Geometry: final body of the model. Coordinates: model frame, mm. Give positions to 0.01 mm unless a question says otherwise; leave off trailing zeros. Write each loop counter-clockwise with the first axis right and the second up, starting at its lowest first coordinate (ties: lowest second). Pieces come first, ordered by that corner, then holes. Notation, with made-up numbers: M -33,25.25 L 18,25.25 A23 cw 18,33.25 Z; hole C 9.5,-22.5 d7. An arc over 180 degrees is marked long. Use a Markdown table: item, result. Add a question column.
1) Pin query (flat end, axial travel): pin 1 (1.3 mm diameter, centred on x = -10.94, y = -4.36, fed in from -Z) (3 decimals). Return the tip coordinate at first contact, or that it passes through.
2) Section D-D on y = -1.5. Return the cut outline in (x, z), then the cut area to 3 significant figures.
3) Section C-C on x = -6. Return the cut outline in (y, z).
4) Line query: line 1 (Y direction, x = -10.5, z = 0.15); line 2 (Y direction, x = -5, z = 1.5); line 3 (X direction, y = -2.75, z = 0.25). Output: solid intervals per line, ascending.
5) Section B-B on z = 2.45. Return the cut outline in (x, y), then the cut area to 3 significant figures.
6) Section A-A on x = -10.5. Return the cut outline in (y, z).
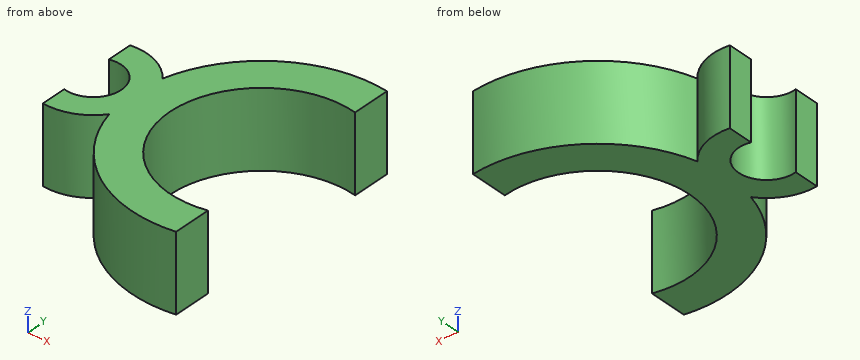
```python
from build123d import *

# Parameters (mm, degrees)
F1_DEPTH = 3


with BuildPart() as f1:
    # F0 (on Top) → F1 (new body)
    with BuildSketch(Plane.XY):
        with BuildLine():
            ThreePointArc((-3.568038, -7.869875), (-7.935237, -4.352574), (-3.568038, -0.835273))
            Line((-3.568038, -0.835273), (-3.568038, 0.689391))
            ThreePointArc((-3.568038, 0.689391), (-7.146301, -0.097234), (-9.273883, -3.079873))
            ThreePointArc((-9.273883, -3.079873), (-10.131319, -2.418957), (-11.20402, -2.272952))
            Line((-11.20402, -2.272952), (-11.20402, -3.288286))
            ThreePointArc((-11.20402, -3.288286), (-9.841317, -4.356456), (-11.20402, -5.424626))
            Line((-11.20402, -5.424626), (-11.20402, -6.439959))
            ThreePointArc((-11.20402, -6.439959), (-10.13018, -6.293478), (-9.272384, -5.631078))
            ThreePointArc((-9.272384, -5.631078), (-7.1438, -8.609565), (-3.568038, -9.394538))
            Line((-3.568038, -9.394538), (-3.568038, -7.869875))
        make_face()
    extrude(amount=F1_DEPTH)


solid = f1.part
```
Found:
| question | item | result |
|---|---|---|
| 1 | pin 1 | through |
| 2 | outline | M -8.56,0 L -6.53,0 L -6.53,3 L -8.56,3 Z |
| 2 | area | 6.09 mm² |
| 3 | outline | M -9.17,0 L -7.54,0 L -7.54,3 L -9.17,3 Z; M -1.16,0 L 0.47,0 L 0.47,3 L -1.16,3 Z |
| 4 | line 1 | -6.41 to -5.36, -3.35 to -2.3 |
| 4 | line 2 | -9.41 to -7.89, -0.81 to 0.7 |
| 4 | line 3 | -11.2 to -9.59, -9.18 to -7.56 |
| 5 | outline | M -11.2,-6.44 A2.1 ccw -9.27,-5.63 A5.1 ccw -3.57,-9.39 L -3.57,-7.87 A3.6 cw long -3.57,-0.84 L -3.57,0.69 A5.1 ccw -9.27,-3.08 A2.1 ccw -11.2,-2.27 L -11.2,-3.29 A1.1 cw long -11.2,-5.42 Z |
| 5 | area | 27.3 mm² |
| 6 | outline | M -6.41,0 L -5.36,0 L -5.36,3 L -6.41,3 Z; M -3.35,0 L -2.3,0 L -2.3,3 L -3.35,3 Z |
